Input: part model. Units: mm. Frame: model coordinates. Face numbers are marked on the shaded views. Give positions to 0.01 mm unless a question says otherwise; leave off trailing zeros. Loops run counter-clockwise (first coordinate to the right, second up) from the corner with the lowest first, then second, coordinate; pieces in that order, holes last.
Autodesk Inventor part; units mm, degrees
ref_plane "YZ Plane" through (0, 0, 0) normal (1, 0, 0) x (0, 1, 0)
ref_plane "XZ Plane" through (0, 0, 0) normal (0, 1, 0) x (-1, 0, 0)
ref_plane "XY Plane" through (0, 0, 0) normal (0, 0, 1) x (1, 0, 0)
sketch "Sketch1" plane through (0, 0, 0) normal (0, 1, 0) x (-1, 0, 0)
  circle A0 centre (0, 0) radius 14
  dimension "d0" = 28
extrude "Extrusion1" add sketch "Sketch1" along normal blind 1.5
sketch "Sketch2" plane through (0, 0, 0) normal (0, -1, 0) x (1, 0, 0)
  circle A0 centre (0, 0) radius 11
  dimension "d3" = 22
extrude "Extrusion2" add sketch "Sketch2" along normal blind 1.8
sketch "Sketch3" plane through (0, -1.8, 0) normal (0, -1, 0) x (1, 0, 0)
  circle A0 centre (0, 0) radius 12.5
  dimension "d6" = 25
extrude "Extrusion3" add sketch "Sketch3" along normal blind 5.2
chamfer "Chamfer1" distance 1 angle 45 2 edges at (-12.5, -1.8, 0) (-12.5, -7, 0)
thread "Thread1"
sketch "Sketch4" plane through (0, 0, 0) normal (0, 0, 1) x (1, 0, 0)
  line L0 (0, 11.1309) -> (0, -17.3821)
  line L1 (14, 1.5) -> (-14, 1.5)
  circle A0 centre (0, -36.45) radius 40.45
  line L2 (11.5, -7) -> (-11.5, -7)
  point P0 (0, 0)
  point P1 (0, 4)
  point P2 (0, 1.5)
  dimension "d15" = 11
revolve "Revolution1" add sketch "Sketch4" angle 360 about axis through (0, 11.1309, 0) along (0, -1, 0) picked at (7.8142, 1.9608) contours A0 L1 L0
sketch "Sketch5" plane through (0, 0, 0) normal (0, 0, 1) x (1, 0, 0)
  line L0 (-0.75, 5.2944) -> (-0.75, 2.6153)
  line L1 (-0.75, 2.6153) -> (0.75, 2.6153)
  line L2 (0.75, 2.6153) -> (0.75, 5.2944)
  line L3 (0.75, 5.2944) -> (-0.75, 5.2944)
  line L4 (-0.75, 5.2944) -> (0.75, 2.6153) construction
  line L5 (-0.75, 2.6153) -> (0.75, 5.2944) construction
  point P0 (0, 0)
  point P1 (0, 3.9548)
  dimension "d17" = 1.5
extrude "Extrusion4" cut sketch "Sketch5" against normal mid plane 20
sketch "Sketch6" plane through (0, -7, 0) normal (0, -1, 0) x (1, 0, 0)
  circle A0 centre (0, 0) radius 10
  dimension "d20" = 20
extrude "Extrusion5" cut sketch "Sketch6" against normal blind 7.5
chamfer "Chamfer2" distance 0.5 angle 45 2 edges at (-10, 0.5, 0) (-10, -7, 0)
properties part number "Cartridge Glans Cover RS 406-9413 LAPP"
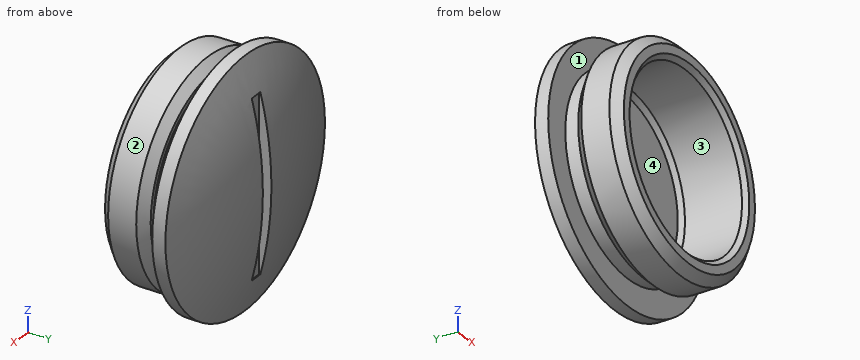
(1) Ray query, probe 1 along Z at (x, y) = (0, -1.25); probe 2 along Z at (x, y) = (0, -3.75); probe 3 along X at (y, z) = (-0.25, 6.5). Return the intervals inside material, ascending.
Values follow:
probe 1: z = -11 to -10, 10 to 11
probe 2: z = -12.5 to -10, 10 to 12.5
probe 3: x = -8.87 to -7.6, 7.6 to 8.87
(2) Cut plane A-A (z = 0). Return the cut outline in (x, y), and give its area (3 significant figures).
Values follow:
outline: (-14, 0) - (-11, 0) - (-11, -1.8) - (-11.5, -1.8) - (-12.5, -2.8) - (-12.5, -6) - (-11.5, -7) - (-10.5, -7) - (-10, -6.5) - (-10, 0) - (-9.5, 0.5) - (9.5, 0.5) - (10, 0) - (10, -6.5) - (10.5, -7) - (11.5, -7) - (12.5, -6) - (12.5, -2.8) - (11.5, -1.8) - (11, -1.8) - (11, 0) - (14, 0) - (14, 1.5) arc R40.45 ccw to (0.75, 3.99) - (0.75, 2.62) - (-0.75, 2.62) - (-0.75, 3.99) arc R40.45 ccw to (-14, 1.5) - close
area: 104 mm2
(3) Cut plane D-D (y = 1). Return the cut outline in (x, z), and give its area (3 significant figures).
Values follow:
outline: circle Ø28 at (0, 0)
area: 616 mm2
(4) Mould query, pull axis Z, two halves, no side actions, for the marked faces 1, 2, 3 and 4. Classes: +Z half, -Z half, draft (parallel to the pull), parting line (faces both ways), or undercut.
Values follow:
face 1: draft
face 2: parting line
face 3: undercut
face 4: undercut
(5) Pin query (flat end, axial travel): pin 1 Ø6 at (x, z) = (-8.5, 8.5) entering from +Y; pin 2 Ø3 at (x, y) = (2, 0.5) entering from +Z; pin 3 Ø6 at (x, z) = (-11, -7.5) entering from +Y. Return the tip coordinate at first contact, or that it passes through.
Values follow:
pin 1: stops at y = 2.98
pin 2: stops at z = 13.99
pin 3: stops at y = 2.66
(6) Cut plane B-B (x = 0). Return the cut outline in (y, z), and give its area (3 significant figures).
Values follow:
outline: (-7, -11.5) - (-6, -12.5) - (-2.8, -12.5) - (-1.8, -11.5) - (-1.8, -11) - (0, -11) - (0, -14) - (1.5, -14) arc R40.45 ccw to (2.74, -10) - (2.62, -10) - (2.62, 10) - (2.74, 10) arc R40.45 ccw to (1.5, 14) - (0, 14) - (0, 11) - (-1.8, 11) - (-1.8, 11.5) - (-2.8, 12.5) - (-6, 12.5) - (-7, 11.5) - (-7, 10.5) - (-6.5, 10) - (0, 10) - (0.5, 9.5) - (0.5, -9.5) - (0, -10) - (-6.5, -10) - (-7, -10.5) - close
area: 87.2 mm2
(7) Cut plane C-C (y = -1). Return the cut outline in (x, z), and give its area (3 significant figures).
Values follow:
outline: circle Ø22 at (0, 0); hole circle Ø20 at (0, 0)
area: 66.0 mm2
